```python
from build123d import *

# Parameters (mm, degrees)
F0_W        = 20
F0_H        = 35
F1_DEPTH    = 15
F2_SIZE     = 15
F3_R        = 2.5
F4_DEPTH    = 20.001
F5_W        = 20
F5_H        = 15
F6_DEPTH    = 20
F7_R        = 2.5
F8_DEPTH    = 20.001
F9_T1_DEPTH = 15


# Not quite as in the source:
# - a fillet or chamfer that OpenCascade refuses, or shapes differently, is made with other operations: its cross-section is extruded or revolved along the edge and cut away or added


with BuildPart() as f1:
    # F0 (on Front) → F1 (new body)
    with BuildSketch(Plane.XZ):
        with Locations((-10, 32.5)):
            Rectangle(F0_W, F0_H)
        Polygon((0, 15), (0, 0), (226.7650184275, 0), (284.8, 0), (284.8, 15), align=None)
        Polygon((284.8, 0), (226.7650184275, 0), (0, -60.6723820371), (0, -76.2), align=None)
        Polygon((0, -60.6723820371), (0, 0), (0, 15), (-20, 15), (-20, -76.2), (0, -76.2), align=None)
    extrude(amount=F1_DEPTH)

    # F2
    f2_edges = [f1.edges().sort_by_distance(p)[0] for p in [
        (0, -7.5, 15),
    ]]
    chamfer(f2_edges, length=F2_SIZE)

    # F3 (on face) → F4 (cut, through all)
    with BuildSketch(Plane.YZ):
        with Locations((-7.5, 40)):
            Circle(F3_R)
    extrude(amount=-F4_DEPTH, mode=Mode.SUBTRACT)

    # F5 (on face) → F6 (join)
    with BuildSketch(Plane(origin=(0, 0, -76.2), x_dir=(1, 0, 0), z_dir=(0, 0, -1))):
        with Locations((-10, 7.5)):
            Rectangle(F5_W, F5_H)
    extrude(amount=F6_DEPTH)

    # F7 (on face) → F8 (cut, through all)
    with BuildSketch(Plane.YZ):
        with Locations((-7.5, -86.2)):
            Circle(F7_R)
    extrude(amount=-F8_DEPTH, mode=Mode.SUBTRACT)

    # F9: fillet of radius 38.1 on 2 edges, made by hand

    # F9_s2 → F9_t1 (join)
    with BuildSketch(Plane.XZ):
        with BuildLine():
            ThreePointArc((0, -11.038341962), (14.9006475381, -41.2608508809), (47.9475089423, -47.8437297148))
            Line((47.9475089423, -47.8437297148), (0, -60.6723820371))
            Line((0, -60.6723820371), (0, -11.038341962))
        make_face()
        with BuildLine():
            ThreePointArc((0, -38.1), (11.1592316368, -11.1592316368), (38.1, 0))
            Line((38.1, 0), (0, 0))
            Line((0, 0), (0, -38.1))
        make_face()
    extrude(amount=F9_T1_DEPTH)


solid = f1.part
```
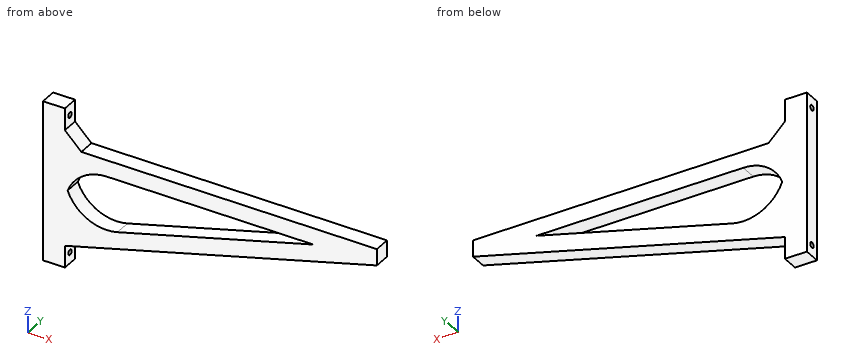
The listing builds one solid part. Answer for the finished solid, in the listing's coordinates (mm). Round coordinates to 2 decimals unless told otherwise and drop trailing zeros. Loops run counter-clockwise (first coordinate to the right, second up) from the corner with the lowest first, then second, coordinate; pieces in that order, holes last. Notation, with made-up numbers: (85, -31) - (105, -31) arc R34 cw to (105, 5) - close; hole circle Ø5 at (-8.5, 3.5). An arc over 180 degrees is marked (long way). Return JSON: item names as keys, results as strings. Group by question number.
1. The part is cut by section D-D on z = -56. Determine the outline of the cut face in (x, y), then the cut area to 3 significant figures.
2. Each of these flat-tipped pins is pushed along its axis until it touches: P1, Ø3, axis at y = -3.5, z = 24, coming from the +X side; P2, Ø4.5, axis at y = -4, z = 37, coming from the +X side; P3, Ø1, axis at x = 138, y = -10, coming from the +Z side; P4, Ø5, axis at x = 97.5, z = 14.5, coming from the +Y side. Where does it stop, or does it pass through?
3. The part is cut by section A-A on y = -7.5. Determine the outline of the cut face in (x, z).
4. The part is cut by section B-B on z = -7. Determine the outline of the cut face in (x, y).
5. Consider probe 1 along Z at (x, y) = (-6.5, -7.5); probe 2 along Z at (x, y) = (99, -9.25); probe 3 along Z at (x, y) = (19.5, -8.5). Determine where each line is inside the solid, lowest interval first.
6. The part is cut by section C-C on x = 59. Determine the outline of the cut face in (y, z).
Resolved:
{
 "1": {"outline": "(-20, -15) - (75.5, -15) - (75.5, 0) - (-20, 0) - close", "area": "1,430 mm²"},
 "2": {"P1": "stops at x = 7.5", "P2": "stops at x = 0", "P3": "stops at z = 15", "P4": "stops at y = 0"},
 "3": {"outline": "(-20, -96.2) - (0, -96.2) - (0, -88.7) - (-20, -88.7) - close; (-20, -83.7) - (0, -83.7) - (0, -76.2) - (284.8, 0) - (284.8, 15) - (15, 15) - (0, 30) - (0, 37.5) - (-20, 37.5) - close; (-20, 42.5) - (0, 42.5) - (0, 50) - (-20, 50) - close; hole (2.48, -24.57) arc R38.1 ccw to (47.95, -47.84) - (226.77, 0) - (38.1, 0) arc R38.1 ccw to start"},
 "4": {"outline": "(-20, -15) - (16.09, -15) - (16.09, 0) - (-20, 0) - close; (200.6, -15) - (258.64, -15) - (258.64, 0) - (200.6, 0) - close"},
 "5": {"probe 1": "z = -96.2 to -88.7, -83.7 to 37.5, 42.5 to 50", "probe 2": "z = -49.71 to -34.18, 0 to 15", "probe 3": "z = -70.98 to -44.29, -4.85 to 15"},
 "6": {"outline": "(-15, -60.41) - (0, -60.41) - (0, -44.89) - (-15, -44.89) - close; (-15, 0) - (0, 0) - (0, 15) - (-15, 15) - close"}
}
